The listing builds one solid part. Answer for the finished solid, in the listing's coordinates (mm). A direction names the side the tool comes from. Coordinates: 2 decimals unless noted, no trailing zeros. Order: outer loops, then holes, each group sorted by start corner. A loop starts at its lowest first (then second) coordinate and runs counter-clockwise, first axis right, second up. Notation, with made-up numbers: (84, -24) -> (94, -24) arc R12 ccw to (94, -13) -> close; hole circle Ø4 at (69, 13). An arc over 180 degrees is marked (long way). Return JSON: item names as keys, results as strings.
```python
from build123d import *

# Parameters (mm, degrees)
F0_R     = 11
F0_W     = 50
F0_H     = 5
F0_H_2   = 80
F0_R_2   = 7.5
F0_R_3   = 4
F1_DEPTH = 10
F2_DEPTH = 50
F3_R     = 1
F4_DEPTH = 25
F5_DEPTH = 5
F6_DEPTH = 15


with BuildPart() as f1:
    # F0 (on Front) → F1 (new body)
    with BuildSketch(Plane.XZ):
        with BuildLine():
            Line((-25, 115), (-25, 0))
            ThreePointArc((-25, 0), (0, -25), (25, 0))
            Line((25, 0), (25, 115))
            Line((25, 115), (-25, 115))
        make_face()
        Circle(F0_R, mode=Mode.SUBTRACT)
        with Locations((0, 117.5)):
            Rectangle(F0_W, F0_H)
        with Locations((0, 160)):
            Rectangle(F0_W, F0_H_2)
        with Locations((0, 185)):
            Circle(F0_R_2, mode=Mode.SUBTRACT)
        with Locations((0, 185)):
            Circle(F0_R_2)
        with Locations((0, 185)):
            Circle(F0_R_3, mode=Mode.SUBTRACT)
        with Locations((0, 185)):
            Circle(F0_R_3)
    extrude(amount=F1_DEPTH)

    # F0 (on Front) → F2 (join)
    with BuildSketch(Plane.XZ):
        with Locations((0, 117.5)):
            Rectangle(F0_W, F0_H)
    extrude(amount=-F2_DEPTH)

    # F3 (on face) → F4 (cut)
    with BuildSketch(Plane.XY.offset(120)):
        with Locations((-12.5, 20)):
            Circle(F3_R)
        with Locations((-12.5, 45)):
            Circle(F3_R)
        with Locations((12.5, 45)):
            Circle(F3_R)
        with Locations((12.5, 20)):
            Circle(F3_R)
    extrude(amount=-F4_DEPTH, mode=Mode.SUBTRACT)

    # F0 (on Front) → F5 (join)
    with BuildSketch(Plane.XZ):
        with Locations((0, 185)):
            Circle(F0_R_2)
        with Locations((0, 185)):
            Circle(F0_R_3, mode=Mode.SUBTRACT)
    extrude(amount=-F5_DEPTH)

    # F0 (on Front) → F6 (join)
    with BuildSketch(Plane.XZ):
        with Locations((0, 185)):
            Circle(F0_R_3)
    extrude(amount=-F6_DEPTH)


solid = f1.part
```
Item 1: The part is cut by section D-D on x = 20.5. Determine the outline of the cut face in (y, z).
Answer list:
{"outline": "(-10, -14.31) -> (0, -14.31) -> (0, 115) -> (50, 115) -> (50, 120) -> (0, 120) -> (0, 200) -> (-10, 200) -> close"}
Item 2: Which of the six approach directions +Z, -Z, +X, -X, +Y, -Y give full straight-line access (tool end or side, diameter ignored) to faces 4 (the flat face through (0, 15, 185)), 5 (the cylindrical face through (-0.976, 2.465, 192.436)), 6 (the flat face through (-25, -2, 100)), 7 (the flat face through (0, 0, 46))?
Answer list:
{"face 4": "+Z, +X, -X, +Y", "face 5": "+Y", "face 6": "+Z, -Z, -X, +Y, -Y", "face 7": "-Z, +X, -X, +Y"}
Item 3: The part is cut by section A-A on x = 0. Determine the outline of the cut face in (y, z).
Answer list:
{"outline": "(-10, -25) -> (0, -25) -> (0, -11) -> (-10, -11) -> close; (-10, 11) -> (0, 11) -> (0, 115) -> (50, 115) -> (50, 120) -> (0, 120) -> (0, 177.5) -> (5, 177.5) -> (5, 181) -> (15, 181) -> (15, 189) -> (5, 189) -> (5, 192.5) -> (0, 192.5) -> (0, 200) -> (-10, 200) -> close"}
Item 4: Determine the mould class of faces 1 (the flat face through (0, -10, 89)), 2 (the cylindrical face through (-0.521, 9.93, 188.966)), 3 (the flat face through (0, 25, 115)) for opening direction Z: pulls with the +Z half, pulls with the -Z half, needs draft (parallel to the pull), parting line crosses it, or undercut.
Answer list:
{"face 1": "needs draft", "face 2": "undercut", "face 3": "pulls with the -Z half"}
Item 5: Find the intervals of material crossed by probe 1 along Y at (x, z) = (-12.5, 118.35); probe 2 along Y at (x, z) = (14, -12); probe 3 along Z at (x, y) = (9, 35), in increasing order.
Answer list:
{"probe 1": "-10 to 19, 21 to 44, 46 to 50", "probe 2": "-10 to 0", "probe 3": "115 to 120"}
Item 6: The part is cut by section B-B on y = 2. Determine the outline of the cut face in (x, z), plus the area to 3 significant figures.
Answer list:
{"outline": "(-25, 115) -> (25, 115) -> (25, 120) -> (-25, 120) -> close; circle Ø15 at (0, 185)", "area": "427 mm2"}
Item 7: Flat-ended cylindrical pins translate along their axes: pin 1 (10 mm diameter, centred on x = 1, y = 27.5, fed in from -Z); pin 2 (20 mm diameter, centred on x = 0, z = 0, fed in from -Y); pin 3 (2.5 mm diameter, centred on x = -12.5, y = 45, fed in from +Z); pin 4 (4.5 mm diameter, centred on x = -1, z = 184.5, fed in from +Y). Find the tip coordinate at first contact, or state that the pin passes through.
Answer list:
{"pin 1": "z = 115", "pin 2": "through", "pin 3": "z = 120", "pin 4": "y = 15"}
Item 8: The part is cut by section C-C on z = 185. Determine the outline of the cut face in (x, y), plus the area to 3 significant figures.
Answer list:
{"outline": "(-25, -10) -> (25, -10) -> (25, 0) -> (7.5, 0) -> (7.5, 5) -> (4, 5) -> (4, 15) -> (-4, 15) -> (-4, 5) -> (-7.5, 5) -> (-7.5, 0) -> (-25, 0) -> close", "area": "655 mm2"}
